```python
from build123d import *

# Parameters (mm, degrees)
SKETCH1_W           = 166.7
SKETCH1_H           = 70
BOSS_EXTRUDE1_DEPTH = 4
SKETCH2_W           = 4
SKETCH2_H           = 70
BOSS_EXTRUDE2_DEPTH = 17
SKETCH3_W           = 20
SKETCH3_H           = 6.8
CUT_EXTRUDE1_DEPTH  = 92.984903653
SKETCH4_W           = 20
SKETCH4_H           = 30
CUT_EXTRUDE2_DEPTH  = 93.807448516
FILLET1_R           = 2
SKETCH5_W           = 20
SKETCH5_H           = 8
CUT_EXTRUDE3_DEPTH  = 93.807448516


with BuildPart() as part:
    # Sketch1 → Boss-Extrude1 (new body)
    with BuildSketch(Plane(origin=(0, 0, 0), x_dir=(1, 0, 0), z_dir=(0, 1, 0))):
        Rectangle(SKETCH1_W, SKETCH1_H)
    extrude(amount=BOSS_EXTRUDE1_DEPTH)

    # Sketch2 → Boss-Extrude2 (add)
    with BuildSketch(Plane(origin=(0, 4, 0), x_dir=(1, 0, 0), z_dir=(0, 1, 0))):
        with Locations((81.35, 0)):
            Rectangle(SKETCH2_W, SKETCH2_H)
        with Locations((-81.35, 0)):
            Rectangle(SKETCH2_W, SKETCH2_H)
    extrude(amount=BOSS_EXTRUDE2_DEPTH)

    # Sketch3 → Cut-Extrude1 (cut, through all)
    with BuildSketch(Plane(origin=(0, 4, 0), x_dir=(1, 0, 0), z_dir=(0, 1, 0))):
        with Locations((-44.35, 11.6)):
            Rectangle(SKETCH3_W, SKETCH3_H)
        with Locations((-44.35, -11.6)):
            Rectangle(SKETCH3_W, SKETCH3_H)
        with Locations((44.35, -11.6)):
            Rectangle(SKETCH3_W, SKETCH3_H)
        with Locations((44.35, 11.6)):
            Rectangle(SKETCH3_W, SKETCH3_H)
    extrude(amount=-CUT_EXTRUDE1_DEPTH, mode=Mode.SUBTRACT)

    # Sketch4 → Cut-Extrude2 (cut, through all)
    with BuildSketch(Plane.XZ):
        Rectangle(SKETCH4_W, SKETCH4_H)
    extrude(amount=-CUT_EXTRUDE2_DEPTH, mode=Mode.SUBTRACT)

    # Fillet1
    fillet1_edges = [part.edges().sort_by_distance(p)[0] for p in [
        (79.35, 4, 0),
        (-79.35, 4, 0),
        (-83.35, 0, 0),
        (83.35, 0, 0),
    ]]
    fillet(fillet1_edges, radius=FILLET1_R)

    # Sketch5 → Cut-Extrude3 (cut, through all)
    with BuildSketch(Plane.XZ):
        with Locations((-21, -31)):
            Rectangle(SKETCH5_W, SKETCH5_H)
        with Locations((-21, 31)):
            Rectangle(SKETCH5_W, SKETCH5_H)
        with Locations((21, 31)):
            Rectangle(SKETCH5_W, SKETCH5_H)
        with Locations((21, -31)):
            Rectangle(SKETCH5_W, SKETCH5_H)
    extrude(amount=-CUT_EXTRUDE3_DEPTH, mode=Mode.SUBTRACT)


solid = part.part
```
The listing builds one solid part. Answer for the finished solid, in the listing's coordinates (mm). A direction names the side the tool comes from. Round coordinates to 2 decimals unless told otherwise and drop trailing zeros. Loops run counter-clockwise (first coordinate to the right, second up) from the corner with the lowest first, then second, coordinate; pieces in that order, holes last. Notation, with made-up numbers: (89, 67.25) - (132, 67.25) arc R7 ccw to (132, 72.25) - close; hole circle Ø10 at (-37.5, 3.5). An arc over 180 degrees is marked (long way). Use one line per item in the form item = value. Start each with the question number.
1. The part is cut by section C-C on y = 13.5. Determine the outline of the cut face in (x, z), then the cut area to 3 significant figures.
2. For a pull along Z with two mould halves and no side action, classify faces 4 (the face through (21, 2, -27)), 5 (the face through (-44, 2, -15)), 6 (the face through (-31, 2, -31)) as pulls with the +Z half, pulls with the -Z half, needs draft (parallel to the pull), parting line crosses it, or undercut.
3. Given pin 1 Ø2 at (x, z) = (0.5, -22) entering from -Y; pin 2 Ø8 at (x, z) = (1.5, -19) entering from +Y; pin 3 Ø3 at (x, y) = (24.5, 2) entering from -Z, each flat-ended and moving along its own axis, determine where each tip first touches the part or whether it passes through.
4. The part is cut by section A-A on z = 5. Determine the outline of the cut face in (x, y), then the cut area to 3 significant figures.
5. The part is cut by section B-B on x = -41. Determine the outline of the cut face in (y, z).
6. The part is cut by section D-D on z = 28.5. Determine the outline of the cut face in (x, y).
7. Consider line 1 (X direction, y = 6.25, z = 17.5); line 2 (Z direction, x = 1, y = 3.5); line 3 (X direction, y = 1.5, z = -29). Determine where each line is inside the solid, lowest interval first. Write a range as [from, to].
8. A tool of negligible diameter and unlimited length cuts with its end or side. For faces 1 (the face through (-31, 2, 31)), 2 (the face through (-54.35, 2, -12)), 3 (the face through (-1, 4, -16)), from which of +Z, -Z, +X, -X, +Y, -Y can it reach the whole face along a straight path? Write none if from no direction.
Geometry check:
q1.outline = (-83.35, -35) - (-79.35, -35) - (-79.35, 35) - (-83.35, 35) - close; (79.35, -35) - (83.35, -35) - (83.35, 35) - (79.35, 35) - close
q1.area = 560 mm^2
q2.face_4 = pulls with the -Z half
q2.face_5 = undercut
q2.face_6 = needs draft
q3.pin_1 = 0
q3.pin_2 = 4
q3.pin_3 = -27
q4.outline = (-83.35, 2) arc R2 ccw to (-81.35, 0) - (-10, 0) - (-10, 4) - (-77.35, 4) arc R2 cw to (-79.35, 6) - (-79.35, 21) - (-83.35, 21) - close; (10, 0) - (81.35, 0) arc R2 ccw to (83.35, 2) - (83.35, 21) - (79.35, 21) - (79.35, 6) arc R2 cw to (77.35, 4) - (10, 4) - close
q4.area = 723 mm^2
q5.outline = (0, -35) - (4, -35) - (4, -15) - (0, -15) - close; (0, -8.2) - (4, -8.2) - (4, 8.2) - (0, 8.2) - close; (0, 15) - (4, 15) - (4, 35) - (0, 35) - close
q6.outline = (-83.35, 2) arc R2 ccw to (-81.35, 0) - (-31, 0) - (-31, 4) - (-77.35, 4) arc R2 cw to (-79.35, 6) - (-79.35, 21) - (-83.35, 21) - close; (-11, 0) - (11, 0) - (11, 4) - (-11, 4) - close; (31, 0) - (81.35, 0) arc R2 ccw to (83.35, 2) - (83.35, 21) - (79.35, 21) - (79.35, 6) arc R2 cw to (77.35, 4) - (31, 4) - close
q7.line_1 = [-83.35, -79.35], [79.35, 83.35]
q7.line_2 = [-35, -15], [15, 35]
q7.line_3 = [-83.29, -31], [-11, 11], [31, 83.29]
q8.face_1 = +Z, +Y, -Y
q8.face_2 = +Y, -Y
q8.face_3 = +Z, -Z, +Y
